Geometry: see drawing. Coordinates: mm, zero at the bounding-box minimum. A direction names the side the tool comes from. Coordinates: 2 decimals unless noted, no trailing zeros. Order: outer loops, then holes, each group sorted by start corner. A loop starts at its lowest first (then second) coordinate and runs counter-clockwise, first axis right, second up. Notation, with made-up numbers: M 12.25,57.25 L 49.25,57.25 A33 ccw 49.25,95.25 Z; hole C 80.5,75 d5. An arc over 180 degrees is marked long. Answer in a Markdown table with one row per item.
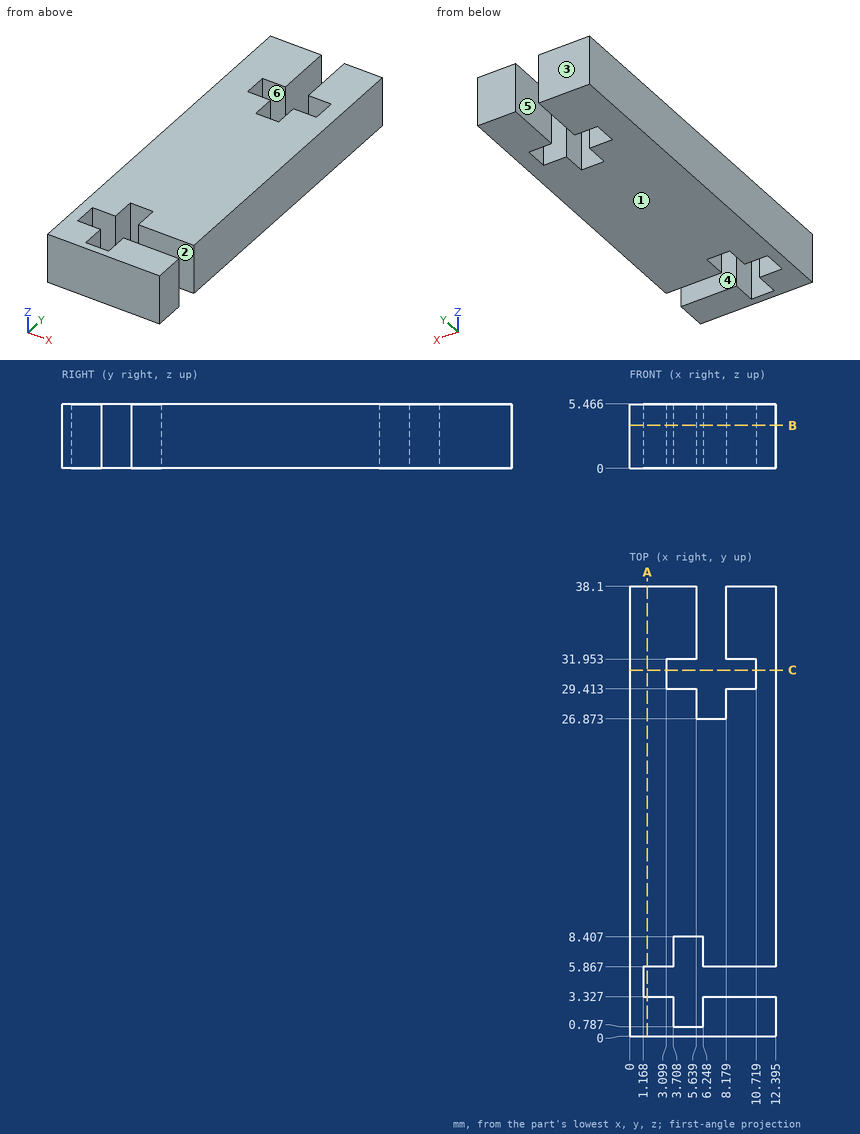
1) Material intervals for probe 1 along Y at (x, z) = (8.5, 0.55); probe 2 along Y at (x, z) = (3.75, 1.85); probe 3 along X at (y, z) = (31, 3.65) (1 decimal), sorted ascending.
Resolved:
| item | result |
|---|---|
| probe 1 | y = 0 to 3.33, 5.87 to 29.41, 31.95 to 38.1 |
| probe 2 | y = 0 to 0.79, 8.41 to 29.41, 31.95 to 38.1 |
| probe 3 | x = 0 to 3.1, 10.7 to 12.4 |
2) Cut plane A-A, the plane x = 1.5. Output: boundary loops of the cut face in (y, z) (1 decimal).
Resolved:
| item | result |
|---|---|
| outline | M 0,0 L 3.3,0 L 3.3,5.5 L 0,5.5 Z; M 5.9,0 L 38.1,0 L 38.1,5.5 L 5.9,5.5 Z |
3) Cut plane C-C, the plane y = 31. Output: boundary loops of the cut face in (x, z) (1 decimal).
Resolved:
| item | result |
|---|---|
| outline | M 0,0 L 3.1,0 L 3.1,5.5 L 0,5.5 Z; M 10.7,0 L 12.4,0 L 12.4,5.5 L 10.7,5.5 Z |
4) Contact query for a flat-ended pin moving along its axis: pin 1 (0.8 mm diameter, centred on x = 7, z = 4, fed in from +Y). Output: stop coordinate, or through.
Resolved:
| item | result |
|---|---|
| pin 1 | stops at y = 26.87 |
5) Mould query, pull axis Y, two halves, no side actions, for the marked faces 1, 2 and 3. Classes: +Y half, -Y half, draft (parallel to the pull), parting line (faces both ways), or undercut.
Resolved:
| item | result |
|---|---|
| face 1 | draft |
| face 2 | undercut |
| face 3 | +Y half |
6) Reachability of the marked faces 4, 5 and 6 from +Z, -Z, +X, -X, +Y, -Y: full face, straight path, thin tool, end or side. Return the list, or none.
Resolved:
| item | result |
|---|---|
| face 4 | +Z, -Z, +X |
| face 5 | +Z, -Z, +Y |
| face 6 | +Z, -Z |
7) Cut plane B-B, the plane z = 3.65. Output: boundary loops of the cut face in (x, y) (1 decimal).
Resolved:
| item | result |
|---|---|
| outline | M 0,0 L 12.4,0 L 12.4,3.3 L 6.2,3.3 L 6.2,0.8 L 3.7,0.8 L 3.7,3.3 L 1.2,3.3 L 1.2,5.9 L 3.7,5.9 L 3.7,8.4 L 6.2,8.4 L 6.2,5.9 L 12.4,5.9 L 12.4,38.1 L 8.2,38.1 L 8.2,32 L 10.7,32 L 10.7,29.4 L 8.2,29.4 L 8.2,26.9 L 5.6,26.9 L 5.6,29.4 L 3.1,29.4 L 3.1,32 L 5.6,32 L 5.6,38.1 L 0,38.1 Z |
